Check sheet for the modelled part. Datum: model origin and axes. Units: mm. A direction names the side the tool comes from. Give positions to 0.01 mm unless a question says otherwise; leave off trailing zeros. Write each loop counter-clockwise with the first axis right and the second up, starting at its lowest first coordinate (ties: lowest second). Pieces come first, ordered by that corner, then holes. Notation, with made-up numbers: M 51.5,27 L 93.5,27 A33 ccw 93.5,66 Z; hole C -13,87 d8. An arc over 180 degrees is marked long. Write item = value, one per line. Start each with the question number.
1) Scan lines: L1, parallel to Z at x = 10.5, y = -2; L2, parallel to X at y = 17.5, z = 15.5; L3, parallel to Y at x = 0, z = 5 (3 decimals). Record each from-to range of solid material in increasing order.
2) Sectioned sample at C-C, the plane x = -15. Record the cut outline in (y, z).
3) Draft check along X on faces 1 (the face through (-3.5, 18, 25)), 2 (the face through (-0.69, -3.1, 10.14)), 3 (the face through (0, -5, 0)). Enter one of: pulls with the +X half, pulls with the -X half, needs draft (parallel to the pull), parting line crosses it, or undercut.
4) Sectioned sample at A-A, the plane z = 23.5. Record the cut outline in (x, y).
5) Sectioned sample at B-B, the plane y = -18. Record the cut outline in (x, z).
6) Gauge pin test, flat ends, axial feed: pin 1 (4 mm diameter, centred on y = -6, z = 15, fed in from -X); pin 2 (8.5 mm diameter, centred on y = 19.5, z = 27, fed in from +X); pin 3 (10 mm diameter, centred on y = 9.5, z = 14, fed in from +X). Record the tip position at first contact, or that the pin passes through.
7) Set-up check for faces 4 (the face through (15, 0, 25)), 5 (the face through (-7.55, -12.96, 24.93)), 6 (the face through (17.74, -6.2, 24.93)), 7 (the face through (0.38, 12.508, 8.464)): record each of +Z, -Z, +X, -X, +Y, -Y from which the full face is reachable in a straight line by a thin tool's end or side.
8) Sectioned sample at D-D, the plane z = 18. Record the cut outline in (x, y) (3 decimals).
from build123d import *
from build123d.topology import SkipClean

# Parameters (mm, degrees)
SKETCH1_R                 = 22.5
BOSS_EXTRUDE1_DEPTH       = 20
CUT_EXTRUDE1_REACH        = 39.583
SKETCH3_R                 = 3.175
F_3_0MM_DOWEL_HOLE1_D     = 3
F_3_0MM_DOWEL_HOLE1_DEPTH = 22
F_3_0MM_DOWEL_HOLE1_TIP   = 0.901290929
BOSS_EXTRUDE3_DEPTH       = 10


with BuildPart() as part:
    # Sketch1 → Boss-Extrude1 (new body)
    with BuildSketch(Plane.XY):
        Circle(SKETCH1_R)
    extrude(amount=BOSS_EXTRUDE1_DEPTH)

    # Sketch3 → Cut-Extrude1 (cut, up to next)
    with BuildSketch(Plane.XY.offset(20), mode=Mode.PRIVATE) as cut_extrude1_sk1:
        Circle(SKETCH3_R)
    cut_extrude1_tool1 = extrude(cut_extrude1_sk1.sketch, amount=-CUT_EXTRUDE1_REACH, mode=Mode.PRIVATE) & part.part
    add(cut_extrude1_tool1.solids().sort_by_distance((0, 0, 20))[0], mode=Mode.SUBTRACT)

    # Ø3.0mm Dowel Hole1
    with Locations(Plane(origin=(0.332625349, 22.497541207, 9.950983977), x_dir=(0.999890720328, -0.014783348841, 0), z_dir=(0.014783348841, 0.999890720328, 0))):
        with Locations((0, 0)):
            Hole(F_3_0MM_DOWEL_HOLE1_D / 2, depth=F_3_0MM_DOWEL_HOLE1_DEPTH)
            with Locations((0, 0, -(F_3_0MM_DOWEL_HOLE1_DEPTH + F_3_0MM_DOWEL_HOLE1_TIP / 2))):  # 118° drill point
                Cone(0, F_3_0MM_DOWEL_HOLE1_D / 2, F_3_0MM_DOWEL_HOLE1_TIP, mode=Mode.SUBTRACT)

    # Sketch6 → Boss-Extrude3 (add)
    with SkipClean():  # the faces are left unmerged after this step: merging them gives an invalid solid
        with BuildSketch(Plane.XY.offset(20)):
            with BuildLine():
                Line((-17.498376555, 14.144144299), (-10.881805097, 10.324064986))
                ThreePointArc((-10.881805097, 10.324064986), (-7.5, 12.990381057), (-3.5, 14.585952146))
                Line((-3.5, 14.585952146), (-3.5, 22.226110771))
                ThreePointArc((-3.5, 22.226110771), (-11.25, 19.485571585), (-17.498376555, 14.144144299))
            make_face()
            with BuildLine():
                Line((14.381805097, 4.26188716), (20.998376555, 8.081966472))
                ThreePointArc((20.998376555, 8.081966472), (22.5, 0), (20.998376555, -8.081966472))
                Line((20.998376555, -8.081966472), (14.381805097, -4.26188716))
                ThreePointArc((14.381805097, -4.26188716), (15, 0), (14.381805097, 4.26188716))
            make_face()
            with BuildLine():
                Line((-3.5, -14.585952146), (-3.5, -22.226110771))
                ThreePointArc((-3.5, -22.226110771), (-11.25, -19.485571585), (-17.498376555, -14.144144299))
                Line((-17.498376555, -14.144144299), (-10.881805097, -10.324064986))
                ThreePointArc((-10.881805097, -10.324064986), (-7.5, -12.990381057), (-3.5, -14.585952146))
            make_face()
        extrude(amount=BOSS_EXTRUDE3_DEPTH)


solid = part.part
Data:
q1.L1 = 0 to 20
q1.L2 = -14.14 to 14.14
q1.L3 = -22.5 to -3.175, 3.175 to 22.5
q2.outline = M -16.77,0 L 16.77,0 L 16.77,30 L 12.7,30 L 12.7,20 L -12.7,20 L -12.7,30 L -16.77,30 Z
q3.face_1 = pulls with the +X half
q3.face_2 = undercut
q3.face_3 = needs draft
q4.outline = M -17.5,-14.14 A22.5 ccw -3.5,-22.23 L -3.5,-14.59 A15 cw -10.88,-10.32 Z; M -17.5,14.14 L -10.88,10.32 A15 cw -3.5,14.59 L -3.5,22.23 A22.5 ccw Z; M 14.38,-4.26 L 21,-8.08 A22.5 ccw 21,8.08 L 14.38,4.26 A15 cw Z
q5.outline = M -13.5,0 L 13.5,0 L 13.5,20 L -3.5,20 L -3.5,30 L -13.5,30 Z
q6.pin_1 = -22.14
q6.pin_2 = -3.5
q6.pin_3 = 22.05
q7.face_4 = +Z, -X
q7.face_5 = +Z, +X
q7.face_6 = +Z, -X, -Y
q7.face_7 = none
q8.outline = C 0,0 d45; hole C 0,0 d6.35
